Model file for the job. Use its own axes, mm. Face numbers are marked on the shaded views. A direction names the side the tool comes from. Give positions to 0.01 mm unless a question says otherwise; leave off trailing zeros. Loops run counter-clockwise (first coordinate to the right, second up) from the corner with the lowest first, then second, coordinate; pieces in that order, holes last. Notation, with made-up numbers: M 75.25,-40 L 94.25,-40 A22 ccw 94.25,-2 Z; hole C 43.25,-29.5 d1. An arc over 180 degrees is marked long. Use CSV: the item, a comma, the result in double quotes. Start each with the question number.
(1) Slice it at B-B on y = 1.5. List the corners of the cut face in (x, z), and give its area (3 significant figures).
(2) Slice it at C-C on z = 0. List the corners of the cut face in (x, y).
(3) Two-plate mould, pull along Y, no slides. Class the marked faces 1, 2 and 3: pulls with the +Y half, pulls with the -Y half, needs draft (parallel to the pull), parting line crosses it, or undercut.
(4) Wall check: line 1 along X through (y, z) = (4.5, -13); line 2 along Y through (x, z) = (-3, 0); line 3 along Z through (x, y) = (0, 5). Give the ranges that are in metal, low to high. Write a range as from..to.
(5) Slice it at A-A on x = 0. List the corners of the cut face in (y, z).
(6) Tool access for the marked faces 4 and 5: list every direction of +Z, -Z, +X, -X, +Y, -Y with a clear straight run to the whole face (end or side of a thin tool).
(7) Flat gauge pins, fed straight in: P1, Ø1.5, axis at x = -3, y = 4, coming from the +Z side; P2, Ø1.7, axis at y = 6.5, z = 0.5, coming from the -X side. Where does each tip first touch, or does it go through?
(8) Slice it at D-D on z = 14.5. List the corners of the cut face in (x, y), and give its area (3 significant figures).
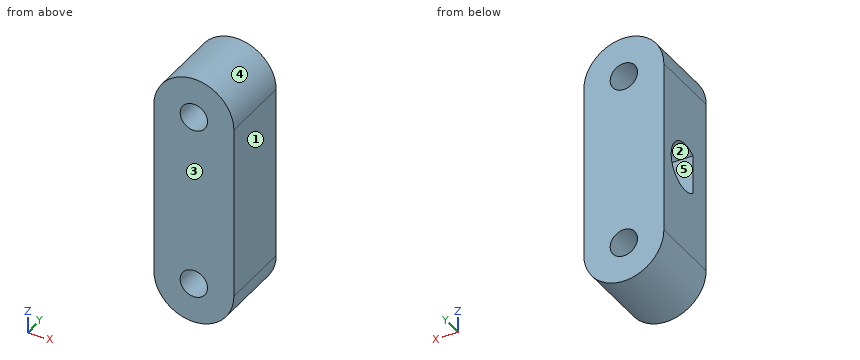
```python
from build123d import *

# Parameters (mm, degrees)
EXTRUDE_1_DEPTH     = 11
SKETCH_2_R          = 2.05
CUT_EXTRUDE_1_DEPTH = 12
SKETCH_3_R          = 3.6
CUT_EXTRUDE_2_DEPTH = 10
EXTRUDE_3_DEPTH     = 10


with BuildPart() as part:
    # 草图1 → 凸台-拉伸1 (new body)
    with BuildSketch(Plane(origin=(0, 0, 0), x_dir=(1, 0, 0), z_dir=(0, 1, 0))):
        with BuildLine():
            Line((-6, -13), (-6, 13))
            ThreePointArc((-6, 13), (0, 19), (6, 13))
            Line((6, 13), (6, -13))
            ThreePointArc((6, -13), (0, -19), (-6, -13))
        make_face()
    extrude(amount=EXTRUDE_1_DEPTH)

    # 草图2 → 切除-拉伸1 (cut, through all)
    with BuildSketch(Plane(origin=(0, 11, 0), x_dir=(1, 0, 0), z_dir=(0, 1, 0))):
        with Locations((0, 13)):
            Circle(SKETCH_2_R)
        with Locations((0, -13)):
            Circle(SKETCH_2_R)
    extrude(amount=-CUT_EXTRUDE_1_DEPTH, mode=Mode.SUBTRACT)

    # 草图3 → 切除-拉伸2 (cut)
    with BuildSketch(Plane.ZY.offset(6)):
        with Locations((0, 5.5)):
            Circle(SKETCH_3_R)
    extrude(amount=-CUT_EXTRUDE_2_DEPTH, mode=Mode.SUBTRACT)

    # 草图4 → 凸台-拉伸3 (add)
    with BuildSketch(Plane.ZY.offset(6)):
        with BuildLine():
            Line((2.959307351, 3.45), (-2.959307351, 3.45))
            ThreePointArc((-2.959307351, 3.45), (0, 1.9), (2.959307351, 3.45))
        make_face()
    extrude(amount=-EXTRUDE_3_DEPTH)


solid = part.part
```
Reply:
1,outline,"M -6,-13 A6 ccw 6,-13 L 6,13 A6 ccw -6,13 Z; hole C 0,-13 d4.1; hole C 0,13 d4.1"
1,area,"399 mm^2"
2,outline,"M -6,0 L 6,0 L 6,11 L -6,11 L -6,9.1 L 4,9.1 L 4,3.45 L -6,3.45 Z"
3,face 1,"needs draft"
3,face 2,"undercut"
3,face 3,"pulls with the -Y half"
4,line 1,"x = -6..-2.05, 2.05..6"
4,line 2,"y = 0..3.45, 9.1..11"
4,line 3,"z = -19..-15.05, -10.95..-3.57, 3.57..10.95, 15.05..19"
5,outline,"M 0,-19 L 11,-19 L 11,-15.05 L 0,-15.05 Z; M 0,-10.95 L 11,-10.95 L 11,10.95 L 0,10.95 Z; M 0,15.05 L 11,15.05 L 11,19 L 0,19 Z; hole M 3.45,-2.96 A3.6 ccw long 3.45,2.96 Z"
6,face 4,"+Z, +Y, -Y"
6,face 5,"-X"
7,P1,"stops at z = 18.56"
7,P2,"stops at x = 4"
8,outline,"M -5.81,0 L -1.4,0 L -1.4,11 L -5.81,11 Z; M 1.4,0 L 5.81,0 L 5.81,11 L 1.4,11 Z"
8,area,"97.1 mm^2"
